Model file for the job. Use its own axes, mm. A direction names the side the tool comes from. Coordinates: 2 decimals unless noted, no trailing zeros. Loops run counter-clockwise (first coordinate to the right, second up) from the corner with the lowest first, then second, coordinate; pieces in that order, holes last. Notation, with made-up numbers: (34, -8.5) -> (64, -8.5) arc R21 ccw to (64, 25.5) -> close; hole circle Ø5 at (10.25, -35). An arc over 180 degrees is marked (long way). Use one line per item in the form item = value.
```python
from build123d import *

# Parameters (mm, degrees)
F1_DEPTH  = 7.5
F2_R      = 3.2
F3_DEPTH  = 15.001
F5_DEPTH  = 2.7
F7_DEPTH  = 5.9
F8_R      = 3.2
F9_DEPTH  = 15.001
F11_DEPTH = 2.7
F12_R     = 3.2
F13_DEPTH = 15.001
F16_DEPTH = 5.4
F17_W     = 80
F17_H     = 15
F18_DEPTH = 4
F19_R     = 3.2
F20_DEPTH = 13
F21_R     = 3.2
F22_DEPTH = 4


with BuildPart() as f1:
    # F0 (on Front) → F1 (new body, symmetric)
    with BuildSketch(Plane.XZ):
        Polygon((-69, 0), (0, 0), (0, 15), (-80, 15), (-80, 11), align=None)
    extrude(amount=F1_DEPTH, both=True)

    # F2 (on face) → F3 (cut, through all)
    with BuildSketch(Plane.XY.offset(15)):
        with Locations((-12, 0)):
            Circle(F2_R)
    extrude(amount=-F3_DEPTH, mode=Mode.SUBTRACT)

    # F4 (on Front) → F5 (cut, symmetric)
    with BuildSketch(Plane.XZ):
        Polygon((-26.9977786002, 4.1), (-23.9955572004, 9.3), (-23.9955572004, 15), (-36.0044427996, 15), (-36.0044427996, 9.3), (-33.0022213998, 4.1), align=None)
    extrude(amount=F5_DEPTH, both=True, mode=Mode.SUBTRACT)

    # F6 (on face) → F7 (cut)
    with BuildSketch(Plane.XY.offset(15)):
        Polygon((-15.0022213998, -5.2), (-8.9977786002, -5.2), (-5.9955572004, 0), (-8.9977786002, 5.2), (-15.0022213998, 5.2), (-18.0044427996, 0), align=None)
    extrude(amount=-F7_DEPTH, mode=Mode.SUBTRACT)

    # F8 (on face) → F9 (cut, through all)
    with BuildSketch(Plane.XZ.offset(7.5)):
        with Locations((-30, 9.3)):
            Circle(F8_R)
    extrude(amount=-F9_DEPTH, mode=Mode.SUBTRACT)

    # F10 (on Front) → F11 (cut, symmetric)
    with BuildSketch(Plane.XZ):
        Polygon((-50, 2.4911144009), (-44.8, 5.4933358006), (-44.8, 11.4977786002), (-44.8, 15), (-55.2, 15), (-55.2, 11.4977786002), (-55.2, 5.4933358006), align=None)
    extrude(amount=F11_DEPTH, both=True, mode=Mode.SUBTRACT)

    # F12 (on face) → F13 (cut, through all)
    with BuildSketch(Plane.XZ.offset(7.5)):
        with Locations((-50, 8.4955572004)):
            Circle(F12_R)
    extrude(amount=-F13_DEPTH, mode=Mode.SUBTRACT)

    # F15 (on offset) → F16 (cut)
    with BuildSketch(Plane(origin=(-31.6715728753, 0, -31.6715728753), x_dir=(0.7071067812, 0, -0.7071067812), z_dir=(-0.7071067812, 0, -0.7071067812))):
        Polygon((-48.3422742884, 0), (-51.3444956882, 5.2), (-57.3489384878, 5.2), (-66.0035713375, 5.2), (-66.0035713375, -5.2), (-57.3489384878, -5.2), (-51.3444956882, -5.2), align=None)
    extrude(amount=-F16_DEPTH, mode=Mode.SUBTRACT)

    # F17 (on face) → F18 (join)
    with BuildSketch(Plane.XY.offset(15)):
        with Locations((-40, 0)):
            Rectangle(F17_W, F17_H)
    extrude(amount=F18_DEPTH)

    # F19 (on face) → F20 (cut)
    with BuildSketch(Plane(origin=(-34.5, 0, -34.5), x_dir=(0.7071067812, 0, -0.7071067812), z_dir=(-0.7071067812, 0, -0.7071067812))):
        with Locations((-54.346717088, 0)):
            Circle(F19_R)
    extrude(amount=-F20_DEPTH, mode=Mode.SUBTRACT)

    # F21 (on face) → F22 (cut, through all)
    with BuildSketch(Plane.XY.offset(19)):
        with Locations((-12, 0)):
            Circle(F21_R)
    extrude(amount=-F22_DEPTH, mode=Mode.SUBTRACT)


solid = f1.part
```
Q1. Which spindle directions (+Z, -Z, +X, -X, +Y, -Y) get a long thin tool onto all of the face, cutting with end or side? Do faces 4 (the face through (-41, -7.5, 9)), 5 (the face through (-44.8, 0, 10)). Say none if no direction does.
Result:
face_4 = +Z, -Z, +X, -X, -Y
face_5 = none
Q2. Band-saw the part on D-D, the plane x = -12. Write the cut outline in (y, z).
Result:
outline = (-7.5, 0) -> (-3.2, 0) -> (-3.2, 9.1) -> (-5.2, 9.1) -> (-5.2, 15) -> (-3.2, 15) -> (-3.2, 19) -> (-7.5, 19) -> close; (3.2, 0) -> (7.5, 0) -> (7.5, 19) -> (3.2, 19) -> (3.2, 15) -> (5.2, 15) -> (5.2, 9.1) -> (3.2, 9.1) -> close
Q3. Wall check: line 1 along Y through (x, z) = (-32.5, 5.5); line 2 along Z through (x, y) = (-30, -6.35); line 3 along X through (y, z) = (-4.5, 6). Give the ranges that are in metal, low to high.
Result:
line_1 = -7.5 to -2.7, 2.7 to 7.5
line_2 = 0 to 6.1, 12.5 to 19
line_3 = -75 to -69.34, -66.04 to -52, -48 to 0
Q4. Band-saw the part on C-C, the plane y = -4.5. Write the cut outline in (x, z), and give its area (3 significant figures).
Result:
outline = (-80, 11) -> (-69, 0) -> (0, 0) -> (0, 19) -> (-80, 19) -> close; hole (-78.34, 15) -> (-67.69, 4.35) -> (-63.87, 8.17) -> (-70.71, 15) -> close; hole circle Ø6.4 at (-50, 8.5); hole circle Ø6.4 at (-30, 9.3); hole (-15.41, 9.1) -> (-8.59, 9.1) -> (-8.59, 15) -> (-15.41, 15) -> close
area = 1,290 mm2
Q5. Mould opens along Z. For faces 1 (the face through (-41, 0, 19)), 2 (the face through (-49, -2.7, 12)), 3 (the face through (0, 0, 9)) say: released by +Z, released by -Z, zero draft, split by the parting line, or undercut.
Result:
face_1 = released by +Z
face_2 = undercut
face_3 = zero draft
Q6. Pin check, flat tip, straight feed: pin 1 Ø1 at (y, z) = (4, 9.5) entering from -X. Stop position of the tip, or through.
Result:
pin_1 = -79
Q7. Band-saw the part on A-A, the plane x = -30. Write the cut outline in (y, z), and give its area (3 significant figures).
Result:
outline = (-7.5, 0) -> (7.5, 0) -> (7.5, 6.1) -> (2.7, 6.1) -> (2.7, 4.1) -> (-2.7, 4.1) -> (-2.7, 6.1) -> (-7.5, 6.1) -> close; (-7.5, 12.5) -> (-2.7, 12.5) -> (-2.7, 15) -> (2.7, 15) -> (2.7, 12.5) -> (7.5, 12.5) -> (7.5, 19) -> (-7.5, 19) -> close
area = 165 mm2
Q8. Band-saw the part on B-B, the plane z = 17. Write the cut outline in (x, y).
Result:
outline = (-80, -7.5) -> (0, -7.5) -> (0, 7.5) -> (-80, 7.5) -> close; hole circle Ø6.4 at (-12, 0)
